Job drawing, mm, ordinate dimensions from the low corner. One solid piece. Round coordinates to 2 decimals unless told otherwise and drop trailing zeros. Write each loop counter-clockwise with the first axis right and the second up, starting at its lowest first coordinate (ties: lowest second). Pieces come first, ordered by that corner, then holes.
1) Saw through at A-A (z = 2). Write the cut outline in (x, y), plus the area to 3 significant figures.
2) Wall check: probe 1 along X at (y, z) = (4.05, 2); probe 2 along Z at (x, y) = (160.5, 1.25). Give the ranges that are in metal, low to high.
3) Saw through at C-C (x = 78). Write the cut outline in (y, z).
4) Flat gauge pin, fed straight in: pin 1 (1.5 mm diameter, centred on y = 3, z = 1.5, fed in from -X). Where does the tip first touch, or does it go through?
5) Saw through at B-B (y = 2.5). Write the cut outline in (x, z).
6) Pull direction Y, two halves, no side cores. Call the marked faces 1 and 2: +Y half, -Y half, draft (parallel to the pull), parting line (faces both ways), or undercut.
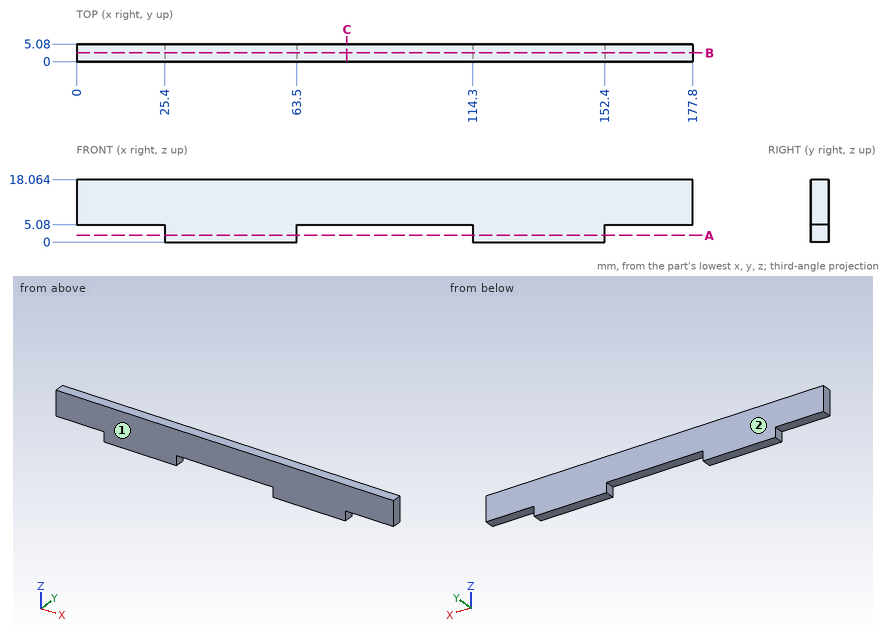
Evaluation:
1. outline: (25.4, 0) - (63.5, 0) - (63.5, 5.08) - (25.4, 5.08) - close; (114.3, 0) - (152.4, 0) - (152.4, 5.08) - (114.3, 5.08) - close
1. area: 387 mm2
2. probe 1: x = 25.4 to 63.5, 114.3 to 152.4
2. probe 2: z = 5.08 to 18.06
3. outline: (0, 5.08) - (5.08, 5.08) - (5.08, 18.06) - (0, 18.06) - close
4. pin 1: stops at x = 25.4
5. outline: (0, 5.08) - (25.4, 5.08) - (25.4, 0) - (63.5, 0) - (63.5, 5.08) - (114.3, 5.08) - (114.3, 0) - (152.4, 0) - (152.4, 5.08) - (177.8, 5.08) - (177.8, 18.06) - (0, 18.06) - close
6. face 1: -Y half
6. face 2: +Y half
